```python
from build123d import *

# Parameters (mm, degrees)
F0_W     = 6
F0_H     = 0.3
F1_DEPTH = 7
F2_R     = 18
F3_DEPTH = 2
F4_R     = 2


# Not quite as in the source:
# - a feature names something its author has since deleted; it is built from what else it names


with BuildPart() as f1:
    # F0 (on Top) → F1 (new body)
    with BuildSketch(Plane.XY):
        with BuildLine():
            ThreePointArc((3.5, -3), (0, -3.3086313325), (-3.5, -3))
            Line((-3.5, -3), (-3.5, -65))
            Line((-3.5, -65), (-23.5, -65))
            Line((-23.5, -65), (-23.5, -70))
            Line((-23.5, -70), (-17.5, -70))
            Line((-17.5, -70), (-3.6, -70))
            Line((-3.6, -70), (-3.6, -67))
            Line((-3.6, -67), (3.6, -67))
            Line((3.6, -67), (3.6, -70))
            Line((3.6, -70), (17.5, -70))
            Line((17.5, -70), (23.5, -70))
            Line((23.5, -70), (23.5, -65))
            Line((23.5, -65), (3.5, -65))
            Line((3.5, -65), (3.5, -3))
        make_face()
        with BuildLine():
            ThreePointArc((20, 16.6913686675), (-12.8452325787, 32.0210783843), (-3.5, -3))
            ThreePointArc((-3.5, -3), (0, -3.3086313325), (3.5, -3))
            ThreePointArc((3.5, -3), (15.3297097168, 3.8461360889), (20, 16.6913686675))
        make_face()
        with Locations((-20.5, -70.15)):
            Rectangle(F0_W, F0_H)
        with Locations((20.5, -70.15)):
            Rectangle(F0_W, F0_H)
    extrude(amount=F1_DEPTH)

    # F2 (on face) → F3 (cut)
    with BuildSketch(Plane.XY.offset(7)):
        with Locations((0, 16.6913686675)):
            Circle(F2_R)
    extrude(amount=-F3_DEPTH, mode=Mode.SUBTRACT)

    # F4
    f4_edges = [f1.edges().sort_by_distance(p)[0] for p in [
        (-3.5, -3, 3.5),
        (3.5, -3, 3.5),
        (23.5, -65, 3.5),
        (-23.5, -65, 3.5),
        (-3.5, -65, 3.5),
        (3.5, -65, 3.5),
        (-23.5, -70.3, 3.5),
        (23.5, -70.3, 3.5),
    ]]
    fillet(f4_edges, radius=F4_R)


solid = f1.part
```
Geometry: final body of the model. Coordinates: model frame, mm. A direction names the side the tool comes from. Round coordinates to 2 decimals unless told otherwise and drop trailing zeros. Order: outer loops, then holes, each group sorted by start corner. A loop starts at its lowest first (then second) coordinate and runs counter-clockwise, first axis right, second up. Notation, with made-up numbers: (82.5, -35) -> (112.5, -35) arc R7 cw to (112.5, -24) -> close; hole circle Ø9 at (-6, -35). An arc over 180 degrees is marked (long way). Use one line per item in the form item = value.
(1) Draft query along X for faces 1 (the face through (22.9, -69.73, 3.55)), 2 (the face through (-3.5, -33, 3)), 3 (the face through (-11, -70, 3)). Return one class per face: pulls with the +X half, pulls with the -X half, needs draft (parallel to the pull), parting line crosses it, or undercut.
Results list:
face_1 = pulls with the +X half
face_2 = pulls with the -X half
face_3 = undercut
(2) First-contact query: pin 1 Ø3.5 at (x, z) = (-14.5, 2.5) entering from +Y; pin 2 Ø4 at (y, z) = (23, 6) entering from +X; pin 3 Ø3.5 at (y, z) = (-21.5, 3.5) entering from -X. Flat tips, straight axial feed; report the tip coordinate or a pass-through.
Results list:
pin_1 = 32.1
pin_2 = 19.53
pin_3 = -3.5
(3) Access query for faces 4 (the face through (4.1, -64.43, 3.55)), 5 (the face through (3.6, -68, 3)), 6 (the face through (-3.9, -0.88, 6.01)), 7 (the face through (-3.91, -3.4, 3.55)). Directions: +Z, -Z, +X, -X, +Y, -Y. A direction counts if a zero-diameter tool reaches every point of the face in a straight line with its end or side. Return the directions, or none.
Results list:
face_4 = +Z, -Z, +X
face_5 = +Z, -Z, -Y
face_6 = +Z
face_7 = +Z, -Z, -X
(4) Section B-B on x = 0. Return loops of the section in (y, z), and give its area (3 significant figures).
Results list:
outline = (-67, 0) -> (36.69, 0) -> (36.69, 7) -> (34.69, 7) -> (34.69, 5) -> (-1.31, 5) -> (-1.31, 7) -> (-67, 7) -> close
area = 654 mm^2
(5) Section C-C on y = -48. Return loops of the section in (x, z).
Results list:
outline = (-3.5, 0) -> (3.5, 0) -> (3.5, 7) -> (-3.5, 7) -> close
(6) Section A-A on z = 3.5. Return loops of the section in (x, y), and give its area (3 significant figures).
Results list:
outline = (-23.5, -68.3) arc R2 ccw to (-21.5, -70.3) -> (-17.5, -70.3) -> (-17.5, -70) -> (-3.6, -70) -> (-3.6, -67) -> (3.6, -67) -> (3.6, -70) -> (17.5, -70) -> (17.5, -70.3) -> (21.5, -70.3) arc R2 ccw to (23.5, -68.3) -> (23.5, -67) arc R2 ccw to (21.5, -65) -> (5.5, -65) arc R2 cw to (3.5, -63) -> (3.5, -4.61) arc R2 cw to (5, -2.67) arc R20 ccw (long way) to (-5, -2.67) arc R2 cw to (-3.5, -4.61) -> (-3.5, -63) arc R2 cw to (-5.5, -65) -> (-21.5, -65) arc R2 ccw to (-23.5, -67) -> close
area = 1,910 mm^2
(7) Ray query, probe 1 along Y at (x, z) = (0, 6.5); probe 2 along X at (y, z) = (-19, 3.75); probe 3 along Z at (x, y) = (0, 25.5). Return the intervals inside material, ascending. Write a range as [from, to].
Results list:
probe_1 = [-67, -1.31], [34.69, 36.69]
probe_2 = [-3.5, 3.5]
probe_3 = [0, 5]
